Verification items for this drawing (mm, ordinates from the low corner). A direction names the side the tool comes from. Round coordinates to 2 decimals unless told otherwise and drop trailing zeros. Order: outer loops, then holes, each group sorted by start corner. A loop starts at its lowest first (then second) coordinate and runs counter-clockwise, first axis right, second up. Notation, with made-up numbers: (-11, 48) - (41, 48) arc R23 cw to (41, 86) - close; hole circle Ø3 at (10.25, 65). An arc over 180 degrees is marked (long way). Return JSON: item names as keys, results as strings. Group by question number.
Q1. Sectioned sample at B-B, the plane y = 2.25. Record the cut outline in (x, z).
Q2. Gauge pin test, flat ends, axial feed: pin 1 Ø5 at (x, y) = (16, 7) entering from +Z; pin 2 Ø5 at (x, y) = (54, 11) entering from +Z; pin 3 Ø4 at (x, z) = (25, 36) entering from +Y. Record the tip position at first contact, or that the pin passes through.
Q3. Tool access check on the marked faces 1 and 2. Record the directions out of +Z, -Z, +X, -X, +Y, -Y that give a thin tool (end or side, any length) a straight path to the whole face; none if there is none.
Q4. Material ranges on line 1 along X through (y, z) = (1.25, 26); line 2 along Z through (x, y) = (35, 2.2); line 3 along X through (y, z) = (5.75, 4), recorded low to high.
Q5. Sectioned sample at A-A, the plane z = 3. Record the cut outline in (x, y).
Q6. Sectioned sample at D-D, the plane z = 31. Record the cut outline in (x, y), then the cut area to 3 significant figures.
Q7. Sectioned sample at C-C, the plane x = 54. Record the cut outline in (y, z), then the cut area to 3 significant figures.
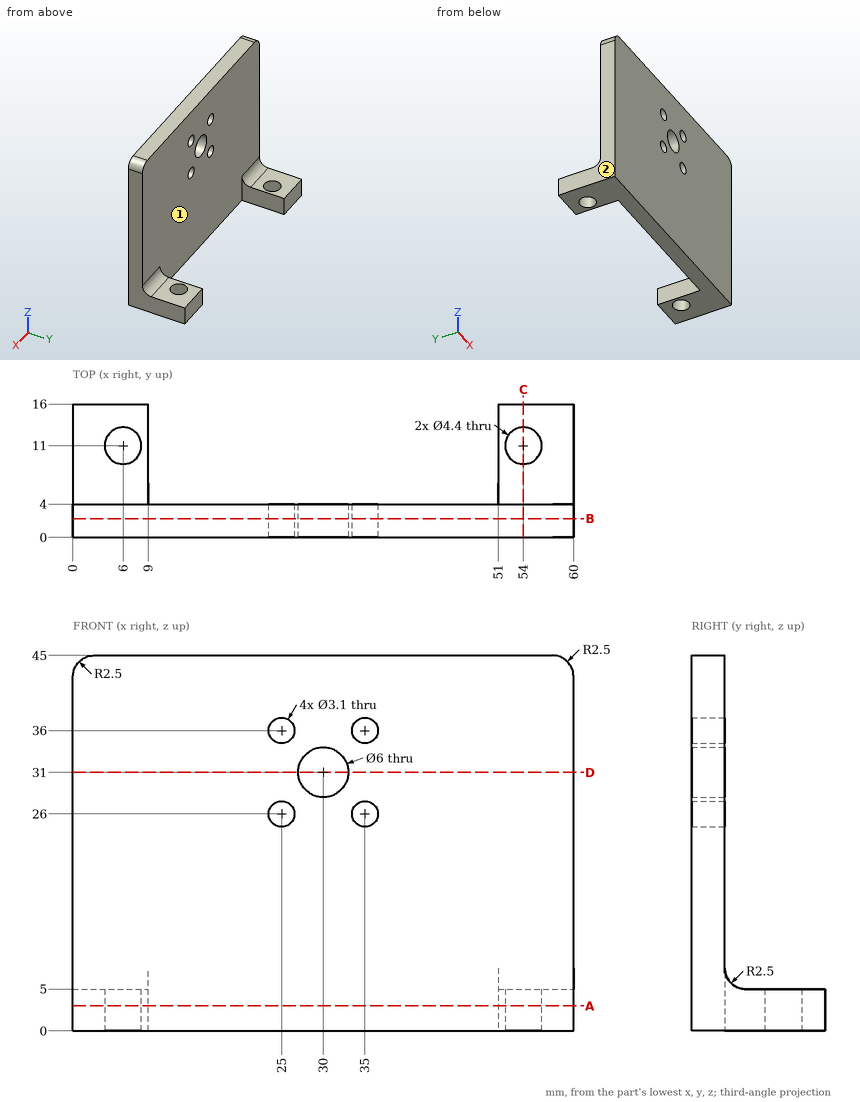
Reply:
{
 "1": {"outline": "(0, 0) - (60, 0) - (60, 42.5) arc R2.5 ccw to (57.5, 45) - (2.5, 45) arc R2.5 ccw to (0, 42.5) - close; hole circle Ø3.1 at (25, 26); hole circle Ø3.1 at (25, 36); hole circle Ø6 at (30, 31); hole circle Ø3.1 at (35, 26); hole circle Ø3.1 at (35, 36)"},
 "2": {"pin 1": "through", "pin 2": "z = 5", "pin 3": "y = 4"},
 "3": {"face 1": "+Z, +Y", "face 2": "+Z, -Z, -X, +Y, -Y"},
 "4": {"line 1": "0 to 23.45, 26.55 to 33.45, 36.55 to 60", "line 2": "0 to 24.45, 27.55 to 34.45, 37.55 to 45", "line 3": "0 to 9, 51 to 60"},
 "5": {"outline": "(0, 0) - (60, 0) - (60, 16) - (51, 16) - (51, 4) - (9, 4) - (9, 16) - (0, 16) - close; hole circle Ø4.4 at (6, 11); hole circle Ø4.4 at (54, 11)"},
 "6": {"outline": "(0, 0) - (27, 0) - (27, 4) - (0, 4) - close; (33, 0) - (60, 0) - (60, 4) - (33, 4) - close", "area": "216 mm^2"},
 "7": {"outline": "(0, 0) - (8.8, 0) - (8.8, 5) - (6.5, 5) arc R2.5 cw to (4, 7.5) - (4, 45) - (0, 45) - close; (13.2, 0) - (16, 0) - (16, 5) - (13.2, 5) - close", "area": "219 mm^2"}
}
